Could you check a few things on this model? Use its own coordinates, in mm. A direction names the side the tool comes from. Round coordinates to 2 decimals unless told otherwise and drop trailing zeros. Loops run counter-clockwise (first coordinate to the right, second up) from the corner with the lowest first, then second, coordinate; pieces in that order, holes last. Notation, with made-up numbers: (-18.5, 24) -> (2.5, 24) arc R17 cw to (2.5, 45) -> close; hole circle Ø10 at (80, 53). An arc over 180 degrees is marked (long way). One line per item, written item: value.
```python
from build123d import *

# Parameters (mm, degrees)
BOSS_EXTRUDE1_DEPTH     = 9
CUT_EXTRUDE1_DEPTH      = 17.347782724
CUT_EXTRUDE1_DEPTH_BACK = 17.347782724
CHAMFER1_SIZE           = 1
FILLET3_R               = 1
SKETCH4_R               = 1.25
CUT_EXTRUDE2_DEPTH      = 17.347782724
CUT_EXTRUDE3_START      = 3
SKETCH5_R               = 2.25
CUT_EXTRUDE3_DEPTH      = 10
FILLET2_R               = 2
CHAMFER2_SIZE           = 1


with BuildPart() as part:
    # Sketch1 → Boss-Extrude1 (new body)
    with BuildSketch(Plane.XY):
        with BuildLine():
            Line((-3.3, 0), (-12, 0))
            Line((-12, 0), (-12, 6.5))
            Line((-12, 6.5), (12, 6.5))
            Line((12, 6.5), (12, 0))
            Line((12, 0), (3.3, 0))
            ThreePointArc((3.3, 0), (0, 3.3), (-3.3, 0))
        make_face()
    extrude(amount=BOSS_EXTRUDE1_DEPTH)

    # Sketch2 → Cut-Extrude1 (cut, two sides: drawn at the far end of the back side and taken through both)
    with BuildSketch(Plane.XY.offset(9).offset(-CUT_EXTRUDE1_DEPTH_BACK)):
        Polygon((-8.355690819, 5), (0, 6.5), (-12, 6.5), (-12, 2.004439372), align=None)
        Polygon((12, 6.5), (0, 6.5), (8.355690819, 5), (12, 2.004439372), align=None)
    extrude(amount=CUT_EXTRUDE1_DEPTH + CUT_EXTRUDE1_DEPTH_BACK, mode=Mode.SUBTRACT)

    # Chamfer1
    chamfer1_edges = [part.edges().sort_by_distance(p)[0] for p in [
        (12, 1.002219686, 9),
        (-12, 1.002219686, 0),
        (-12, 1.002219686, 9),
        (12, 1.002219686, 0),
    ]]
    chamfer(chamfer1_edges, length=CHAMFER1_SIZE)

    # Fillet3
    fillet3_edges = [part.edges().sort_by_distance(p)[0] for p in [
        (12, 0, 4.5),
        (3.3, 0, 4.5),
        (-12, 0, 4.5),
        (-3.3, 0, 4.5),
    ]]
    fillet(fillet3_edges, radius=FILLET3_R)

    # Sketch4 → Cut-Extrude2 (cut, through all)
    with BuildSketch(Plane.XZ):
        with Locations(Location((-5.25, 4.5, 0), (0, 0, 31.315725107))):
            Circle(SKETCH4_R)
        with Locations((5.25, 4.5)):
            Circle(SKETCH4_R)
    extrude(amount=-CUT_EXTRUDE2_DEPTH, mode=Mode.SUBTRACT)

    # Sketch5 → Cut-Extrude3 (cut)
    with BuildSketch(Plane(origin=(0, 0, 0), x_dir=(1, 0, 0), z_dir=(0, 1, 0)).offset(CUT_EXTRUDE3_START)):
        with Locations(Location((-5.25, -4.5, 0), (0, 0, 180))):
            Circle(SKETCH5_R)
        with Locations((5.25, -4.5)):
            Circle(SKETCH5_R)
    extrude(amount=CUT_EXTRUDE3_DEPTH, mode=Mode.SUBTRACT)

    # Fillet2
    fillet2_edges = [part.edges().sort_by_distance(p)[0] for p in [
        (8.355690819, 5, 4.5),
        (-8.355690819, 5, 4.5),
        (0, 6.5, 4.5),
        (-12, 2.004439372, 4.5),
    ]]
    fillet(fillet2_edges, radius=FILLET2_R)

    # Chamfer2
    chamfer2_edges = [part.edges().sort_by_distance(p)[0] for p in [
        (7.591052367, 0, 0),
        (3.562652612, 0.214965561, 0),
        (0, 3.3, 0),
        (-3.562652612, 0.214965561, 0),
        (-7.591052367, 0, 0),
    ]]
    chamfer(chamfer2_edges, length=CHAMFER2_SIZE)
    # the kernel refuses this chamfer: 1 mm, written as the material it takes off along each edge
    with BuildSketch(Plane(origin=(8.758751871, 4.668690619, 0), x_dir=(-0.6347551060767181, -0.7722240167716554, -0.02749587661058638), z_dir=(0.7725160920418075, -0.6349951870183377, 0)), Plane(origin=(-12.986666492, 1.193416171, 0), x_dir=(0.6347551060767181, -0.7722240167716553, -0.02749587661058636), z_dir=(0.7725160920418074, 0.6349951870183378, 0))) as chamfer2_2_piece_1:
        with BuildLine():
            Line((1.028673195, 0), (-0.056547155, -1.027117794))
            Line((-0.056547155, -1.027117794), (-0.076539593, -1.026567876))
            ThreePointArc((-0.076539593, -1.026567876), (-0.034129227, -0.51339783), (-0.019992438, 0.000549918))
            Line((-0.019992438, 0.000549918), (0.000549918, 0.019992438))
            ThreePointArc((0.000549918, 0.019992438), (0.514497665, 0.00585565), (1.029223113, 0.019992438))
            Line((1.029223113, 0.019992438), (1.028673195, 0))
        make_face()
    extrude(amount=5.472914628, mode=Mode.SUBTRACT)
    with BuildSketch(Plane(origin=(7.488761497, 3.123658435, 0), x_dir=(0.6349951870183373, 0.7725160920418078, 0), z_dir=(0.7725160920418078, -0.6349951870183373, 0))) as chamfer2_2_piece_2:
        with BuildLine():
            Line((0.971715729, -0.028284271), (2.028284271, 1.028284271))
            Line((2.028284271, 1.028284271), (2.048284271, 1.028284271))
            ThreePointArc((2.048284271, 1.028284271), (2.02, 0.514142136), (2.02, 0))
            Line((2.02, 0), (2, -0.02))
            ThreePointArc((2, -0.02), (1.485857864, -0.02), (0.971715729, -0.048284271))
            Line((0.971715729, -0.048284271), (0.971715729, -0.028284271))
        make_face()
    revolve(axis=Axis((7.488761497, 3.123658435, 0), (0, 0, 1)), revolution_arc=29.242385329, mode=Mode.SUBTRACT)
    with BuildSketch(Plane(origin=(0.35338761, 6.436560432, 0), x_dir=(-0.176626999834447, -0.9838937339463534, -0.02749587661058635), z_dir=(0.9842658682259174, -0.17669380477391067, 0)), Plane(origin=(-7.842149107, 5.092190171, 0), x_dir=(0.17662699983444718, -0.9838937339463534, -0.027495876610586334), z_dir=(0.9842658682259174, 0.17669380477391086, 0))) as chamfer2_2_piece_3:
        with BuildLine():
            Line((1.028673195, 0), (-0.056547155, -1.027117794))
            Line((-0.056547155, -1.027117794), (-0.076539593, -1.026567876))
            ThreePointArc((-0.076539593, -1.026567876), (-0.034129227, -0.51339783), (-0.019992438, 0.000549918))
            Line((-0.019992438, 0.000549918), (0.000549918, 0.019992438))
            ThreePointArc((0.000549918, 0.019992438), (0.514497665, 0.00585565), (1.029223113, 0.019992438))
            Line((1.029223113, 0.019992438), (1.028673195, 0))
        make_face()
    extrude(amount=7.608474234, mode=Mode.SUBTRACT)
    with BuildSketch(Plane(origin=(0, 4.468028696, 0), x_dir=(0.17669380477391125, 0.9842658682259174, 0), z_dir=(0.9842658682259174, -0.17669380477391125, 0))) as chamfer2_2_piece_4:
        with BuildLine():
            Line((0.971715729, -0.028284271), (2.028284271, 1.028284271))
            Line((2.028284271, 1.028284271), (2.048284271, 1.028284271))
            ThreePointArc((2.048284271, 1.028284271), (2.02, 0.514142136), (2.02, 0))
            Line((2.02, 0), (2, -0.02))
            ThreePointArc((2, -0.02), (1.485857864, -0.02), (0.971715729, -0.048284271))
            Line((0.971715729, -0.048284271), (0.971715729, -0.028284271))
        make_face()
    revolve(axis=Axis((0, 4.468028696, 0), (0, 0, 1)), revolution_arc=20.354484339, mode=Mode.SUBTRACT)
    with BuildSketch(Plane(origin=(-7.488761497, 3.123658435, 0), x_dir=(-0.17669380477391083, 0.9842658682259176, 0), z_dir=(0.9842658682259176, 0.17669380477391083, 0))) as chamfer2_2_piece_5:
        with BuildLine():
            Line((0.971715729, -0.028284271), (2.028284271, 1.028284271))
            Line((2.028284271, 1.028284271), (2.048284271, 1.028284271))
            ThreePointArc((2.048284271, 1.028284271), (2.02, 0.514142136), (2.02, 0))
            Line((2.02, 0), (2, -0.02))
            ThreePointArc((2, -0.02), (1.485857864, -0.02), (0.971715729, -0.048284271))
            Line((0.971715729, -0.048284271), (0.971715729, -0.028284271))
        make_face()
    revolve(axis=Axis((-7.488761497, 3.123658435, 0), (0, 0, 1)), revolution_arc=29.242385329, mode=Mode.SUBTRACT)


solid = part.part
```
(1) For pin 1 Ø3 at (x, y) = (-3, 4) entering from -Z; pin 2 Ø1.3 at (x, z) = (5.5, 4) entering from +Y; pin 3 Ø2 at (y, z) = (5.5, 5.5) entering from -X; pin 4 Ø4 at (x, z) = (5.25, 4.5) entering from +Y, each with a flat end and sliding along its axis, tell me the tip position at first contact or that it passes through.
Results below:
pin 1: stops at z = 0
pin 2: passes through
pin 3: stops at x = -8.96
pin 4: stops at y = 3
(2) We'd pull the mould along X, two halves only. Please class faces 1 (the face through (-4.427, 1.479, 5.44)), 2 (the face through (-2.486, 6.054, 4.944)), 3 (the face through (0, 5.98, 0.51)): +X half, -X half, draft (parallel to the pull), parting line (faces both ways), or undercut.
Results below:
face 1: undercut
face 2: -X half
face 3: parting line
(3) Please list where these lines run through material, in increasing order: L1, parallel to X at y = 2.25, z = 4.5; L2, parallel to Z at x = 5.25, y = 3.7; L3, parallel to X at y = 2.25, z = 3.75.
Results below:
L1: x = -11.61 to -6.5, -4 to -2.41, 2.41 to 4, 6.5 to 11.7
L2: z = 0 to 2.25, 6.75 to 9
L3: x = -11.61 to -6.25, -4.25 to -2.41, 2.41 to 4.25, 6.25 to 11.7
(4) Imagine slicing it at C-C on z = 4.5. Give the number of separate pieces and of enclosed holes in the cut face, then the cut area to 3 significant figures.
Results below:
separate pieces: 3
enclosed holes: 0
area: 65.6 mm²
(5) Imagine slicing it at B-B on x = -5.25. Write out the boundary of the cut face in (y, z), then the cut area to 3 significant figures.
Results below:
outline: (0, 1) -> (1, 0) -> (4.54, 0) -> (5.56, 1) -> (5.56, 2.25) -> (3, 2.25) -> (3, 3.25) -> (0, 3.25) -> close; (0, 5.75) -> (3, 5.75) -> (3, 6.75) -> (5.56, 6.75) -> (5.56, 9) -> (0, 9) -> close
area: 30.0 mm²
(6) Imagine slicing it at D-D on x = -10. Write out the boundary of the cut face in (y, z).
Results below:
outline: (0, 1) -> (1, 0) -> (2.35, 0) -> (3.65, 1) -> (3.65, 9) -> (0, 9) -> close
(7) Imagine slicing it at A-A on z = 1.5. Write out the boundary of the cut face in (x, y).
Results below:
outline: (-12, 1) arc R1 ccw to (-11, 0) -> (-4.18, 0) arc R1 ccw to (-3.21, 0.77) arc R3.3 cw to (3.21, 0.77) arc R1 ccw to (4.18, 0) -> (11, 0) arc R1 ccw to (12, 1) -> (12, 2) -> (8.76, 4.67) arc R2 ccw to (7.84, 5.09) -> (0.35, 6.44) arc R2 ccw to (-0.35, 6.44) -> (-7.84, 5.09) arc R2 ccw to (-8.76, 4.67) -> (-11.27, 2.6) arc R2 ccw to (-12, 1.06) -> close
(8) On a 3-axis mill with a long thin cutter (end or side, diameter ignored), from which of +Z, -Z, +X, -X, +Y, -Y can I reach the whole of each face in a straight line? I mean faces 4 (the face through (10, 3, 0.5)), 5 (the face through (-3.002, 4.145, 4.599)). Say none if no direction works.
Results below:
face 4: -Z, +X, +Y
face 5: +Y
